Autodesk Inventor part; units mm, degrees
ref_plane "YZ Plane" through (0, 0, 0) normal (1, 0, 0) x (0, 1, 0)
ref_plane "XZ Plane" through (0, 0, 0) normal (0, 1, 0) x (-1, 0, 0)
ref_plane "XY Plane" through (0, 0, 0) normal (0, 0, 1) x (1, 0, 0)
sketch "Sketch1" plane through (0, 0, 0) normal (0, 1, 0) x (-1, 0, 0)
  circle A0 centre (0, 0) radius 6.35
  circle A1 centre (0, 0) radius 5.715
  dimension "d0" = 12.7
  dimension "d1" = 0.635
extrude "Extrusion1" add sketch "Sketch1" along normal blind 50.8
sketch "Sketch2" plane through (0, 0, 0) normal (0, -1, 0) x (1, 0, 0)
  circle A0 centre (0, 0) radius 6.35
  circle A1 centre (0, 0) radius 6.35
  circle A2 centre (0, 0) radius 12.065
  dimension "d4" = 24.13
extrude "Extrusion2" add sketch "Sketch2" against normal blind 1.27
sketch "Sketch3" plane through (0, 1.27, 0) normal (0, 1, 0) x (1, 0, 0)
  circle A0 centre (0, 0) radius 12.065
  circle A1 centre (0, 0) radius 12.065
  circle A2 centre (0, 0) radius 12.7
  dimension "d7" = 25.4
extrude "Extrusion3" add sketch "Sketch3" against normal blind 203.2
properties part number "still pipe small.iam" material "Stainless Steel"
Could you check a few things on this model? Use its own coordinates, in mm. A direction names the side the tool comes from. Round coordinates to 2 decimals unless told otherwise and drop trailing zeros. Loops run counter-clockwise (first coordinate to the right, second up) from the corner with the lowest first, then second, coordinate; pieces in that order, holes last. Notation, with made-up numbers: (3.5, 58.25) - (60.5, 58.25) arc R16 ccw to (60.5, 78.25) - close; hole circle Ø3 at (65, -27.5). An arc over 180 degrees is marked (long way). Answer in a Markdown table with one row per item. Add a question column.
(1) I'm going to push flat-ended pins straight in: pin 1 (8 mm diameter, centred on x = 0.5, y = -44.5, fed in from -Z); pin 2 (8 mm diameter, centred on y = 7, z = 2, fed in from +X); pin 3 (12 mm diameter, centred on x = -1.5, y = 22.5, fed in from -Z); pin 4 (1.5 mm diameter, centred on x = 7.5, y = -79.5, fed in from +Z). Where does each tip first touch, or does it pass through?
(2) I need wall thicknesses on line 1 along Z through (x, y) = (0, -100) (3 decimals); line 2 along Z through (x, y) = (0, 17) (3 decimals); line 3 along X through (y, z) = (-19, -0.5). Which ranges of each line are inside material? Lowest first, please.
(3) If we section it at A-A (z = 0): Please give me the cut outline in (x, y) (3 decimals).
(4) If we mould it in two halves opening along X, with no side actions, what happens to faces 4 (the face through (6, 50.8, 1)), 5 (the face through (-5.45, 25.04, -1.72)), 6 (the face through (5.2, 0, 2.9)), 7 (the face through (1.38, 25.69, 6.2))? For each: pulls with the +X half, pulls with the -X half, needs draft (parallel to the pull), parting line crosses it, or undercut.
(5) If we section it at B-B (x = 0): Please give me the cut outline in (y, z) (3 decimals), plus the area to 3 significant figures.
(6) For faces 1 (the face through (3, 1.27, -6)), 2 (the face through (11.51, -99.55, -3.62)), 3 (the face through (-2.75, -98.91, 12.4)), which set-ups out of +Z, -Z, +X, -X, +Y, -Y let a thin tool reach every point of the face, with its end or its side?
(7) If we section it at C-C (y = -145): Please give me the cut outline in (x, z) (3 decimals).
(8) If we section it at D-D (x = -9.5): Please give me the cut outline in (y, z).
Model answer:
| question | item | result |
|---|---|---|
| 1 | pin 1 | stops at z = -12.7 |
| 1 | pin 2 | stops at x = 6.35 |
| 1 | pin 3 | stops at z = -6.35 |
| 1 | pin 4 | stops at z = 10.76 |
| 2 | line 1 | z = -12.7 to -12.065, 12.065 to 12.7 |
| 2 | line 2 | z = -6.35 to -5.715, 5.715 to 6.35 |
| 2 | line 3 | x = -12.69 to -12.05, 12.05 to 12.69 |
| 3 | outline | (-12.7, -201.93) - (-12.065, -201.93) - (-12.065, 0) - (-5.715, 0) - (-5.715, 50.8) - (-6.35, 50.8) - (-6.35, 1.27) - (-12.7, 1.27) - close; (5.715, 0) - (12.065, 0) - (12.065, -201.93) - (12.7, -201.93) - (12.7, 1.27) - (6.35, 1.27) - (6.35, 50.8) - (5.715, 50.8) - close |
| 4 | face 4 | needs draft |
| 4 | face 5 | undercut |
| 4 | face 6 | undercut |
| 4 | face 7 | parting line crosses it |
| 5 | outline | (-201.93, -12.7) - (1.27, -12.7) - (1.27, -6.35) - (50.8, -6.35) - (50.8, -5.715) - (0, -5.715) - (0, -12.065) - (-201.93, -12.065) - close; (-201.93, 12.065) - (0, 12.065) - (0, 5.715) - (50.8, 5.715) - (50.8, 6.35) - (1.27, 6.35) - (1.27, 12.7) - (-201.93, 12.7) - close |
| 5 | area | 337 mm² |
| 6 | face 1 | +Y |
| 6 | face 2 | -Y |
| 6 | face 3 | +Y, -Y |
| 7 | outline | circle Ø25.4 at (0, 0); hole circle Ø24.13 at (0, 0) |
| 8 | outline | (-201.93, -8.43) - (1.27, -8.43) - (1.27, 8.43) - (-201.93, 8.43) - (-201.93, 7.44) - (0, 7.44) - (0, -7.44) - (-201.93, -7.44) - close |
